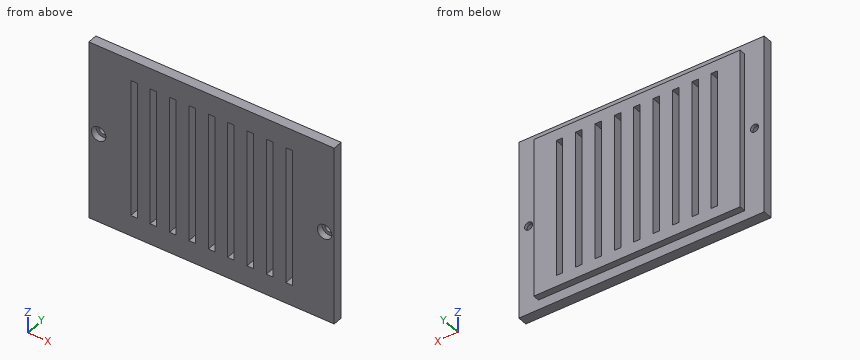
```python
from build123d import *

# Parameters (mm, degrees)
SKETCH1_W           = 76
SKETCH1_H           = 56
BOSS_EXTRUDE1_DEPTH = 3
SKETCH2_W           = 63.9
SKETCH2_H           = 49.9
BOSS_EXTRUDE2_DEPTH = 2
SKETCH3_R           = 2.25
CUT_EXTRUDE1_DEPTH  = 2
CUT_EXTRUDE2_REACH  = 49.466
SKETCH4_R           = 1.25
SKETCH5_W           = 2
SKETCH5_H           = 43
CUT_EXTRUDE3_DEPTH  = 48.465777145


with BuildPart() as part:
    # Sketch1 → Boss-Extrude1 (new body)
    with BuildSketch(Plane(origin=(0, 0, 0), x_dir=(1, 0, 0), z_dir=(0, 1, 0))):
        Rectangle(SKETCH1_W, SKETCH1_H)
    extrude(amount=BOSS_EXTRUDE1_DEPTH)

    # Sketch2 → Boss-Extrude2 (add)
    with BuildSketch(Plane(origin=(0, 3, 0), x_dir=(1, 0, 0), z_dir=(0, 1, 0))):
        Rectangle(SKETCH2_W, SKETCH2_H)
    extrude(amount=BOSS_EXTRUDE2_DEPTH)

    # Sketch3 → Cut-Extrude1 (cut)
    with BuildSketch(Plane.XZ):
        with Locations(Location((-35, 0, 0), (0, 0, 270))):
            Circle(SKETCH3_R)
        with Locations(Location((35, 0, 0), (0, 0, 90))):
            Circle(SKETCH3_R)
    extrude(amount=-CUT_EXTRUDE1_DEPTH, mode=Mode.SUBTRACT)

    # Sketch4 → Cut-Extrude2 (cut, up to next)
    with BuildSketch(Plane.XZ, mode=Mode.PRIVATE) as cut_extrude2_sk1:
        with Locations(Location((-35, 0, 0), (0, 0, 270))):
            Circle(SKETCH4_R)
    cut_extrude2_tool1 = extrude(cut_extrude2_sk1.sketch, amount=-CUT_EXTRUDE2_REACH, mode=Mode.PRIVATE) & part.part
    # Sketch4 → Cut-Extrude2 (cut, up to next)
    with BuildSketch(Plane.XZ, mode=Mode.PRIVATE) as cut_extrude2_sk2:
        with Locations(Location((35, 0, 0), (0, 0, 270))):
            Circle(SKETCH4_R)
    cut_extrude2_tool2 = extrude(cut_extrude2_sk2.sketch, amount=-CUT_EXTRUDE2_REACH, mode=Mode.PRIVATE) & part.part
    add(cut_extrude2_tool1.solids().sort_by_distance((-35, 0, 0))[0], mode=Mode.SUBTRACT)
    add(cut_extrude2_tool2.solids().sort_by_distance((35, 0, 0))[0], mode=Mode.SUBTRACT)

    # Sketch5 → Cut-Extrude3 (cut, through all)
    with BuildSketch(Plane.XZ):
        with Locations((6, 0)):
            Rectangle(SKETCH5_W, SKETCH5_H)
        Rectangle(SKETCH5_W, SKETCH5_H)
        with Locations((12, 0)):
            Rectangle(SKETCH5_W, SKETCH5_H)
        with Locations((18, 0)):
            Rectangle(SKETCH5_W, SKETCH5_H)
        with Locations((24, 0)):
            Rectangle(SKETCH5_W, SKETCH5_H)
        with Locations((-6, 0)):
            Rectangle(SKETCH5_W, SKETCH5_H)
        with Locations((-12, 0)):
            Rectangle(SKETCH5_W, SKETCH5_H)
        with Locations((-18, 0)):
            Rectangle(SKETCH5_W, SKETCH5_H)
        with Locations((-24, 0)):
            Rectangle(SKETCH5_W, SKETCH5_H)
    extrude(amount=-CUT_EXTRUDE3_DEPTH, mode=Mode.SUBTRACT)


solid = part.part
```
Can you work these out from the model? Positions are in its coordinate system, mm. Coordinates: 2 decimals unless noted, no trailing zeros. Order: outer loops, then holes, each group sorted by start corner. A loop starts at its lowest first (then second) coordinate and runs counter-clockwise, first axis right, second up. Notation, with made-up numbers: (84.25, 27) - (101.25, 27) arc R15 cw to (101.25, 38) - close; hole circle Ø5 at (28, 20). An arc over 180 degrees is marked (long way). Answer in a Markdown table with one row per item.
1. Suppose I cut it at A-A (x = 35). Please give me the cut outline in (y, z).
Reply:
| item | result |
|---|---|
| outline | (0, -28) - (3, -28) - (3, -1.25) - (2, -1.25) - (2, -2.25) - (0, -2.25) - close; (0, 2.25) - (2, 2.25) - (2, 1.25) - (3, 1.25) - (3, 28) - (0, 28) - close |
2. Suppose I cut it at C-C (z = 0). Give the number of separate pieces and of enclosed holes in the cut face, and give its area (3 significant figures).
Reply:
| item | result |
|---|---|
| separate pieces | 12 |
| enclosed holes | 0 |
| area | 243 mm^2 |
3. Suppose I cut it at B-B (x = -14). Please give me the cut outline in (y, z), and give its area (3 significant figures).
Reply:
| item | result |
|---|---|
| outline | (0, -28) - (3, -28) - (3, -24.95) - (5, -24.95) - (5, 24.95) - (3, 24.95) - (3, 28) - (0, 28) - close |
| area | 268 mm^2 |
4. If I drill on line 1 along Z through (x, y) = (24, 2); line 2 along Z through (x, y) = (11.5, 4.7); line 3 along Y through (x, z) = (33.5, 21), over which ranges is the centre line in solid material (lowest first)?
Reply:
| item | result |
|---|---|
| line 1 | z = -28 to -21.5, 21.5 to 28 |
| line 2 | z = -24.95 to -21.5, 21.5 to 24.95 |
| line 3 | y = 0 to 3 |
5. For pin 1 (0.6 mm diameter, centred on x = 7.5, y = 4.5, fed in from +Z); pin 2 (3.5 mm diameter, centred on x = -35, z = 0, fed in from +Y); pin 3 (2 mm diameter, centred on x = 35.5, z = 0, fed in from -Y), each with a flat end and sliding along its axis, tell me the tip position at first contact or that it passes through.
Reply:
| item | result |
|---|---|
| pin 1 | stops at z = 24.95 |
| pin 2 | stops at y = 3 |
| pin 3 | stops at y = 2 |
